Input: part model. Units: mm. Frame: model coordinates. Round coordinates to 2 decimals unless told otherwise and drop trailing zeros. Write each loop counter-clockwise with the first axis right and the second up, starting at its lowest first coordinate (ties: lowest second). Pieces come first, ordered by that corner, then holes. Notation, with made-up numbers: (-35, 16.25) -> (-22, 16.25) arc R20 ccw to (-22, 32.25) -> close; hole circle Ø7 at (10.5, -30.75). An arc over 180 degrees is marked (long way). Write item = value, one per line.
```python
from build123d import *

# Parameters (mm, degrees)
SKETCH1_R           = 2.1
BOSS_EXTRUDE1_DEPTH = 3


with BuildPart() as part:
    # Sketch1 → Boss-Extrude1 (new body)
    with BuildSketch(Plane(origin=(0, 0, 0), x_dir=(1, 0, 0), z_dir=(0, 1, 0))):
        with BuildLine():
            Line((65, -70), (-65, -70))
            ThreePointArc((-65, -70), (-98.297426292, -61.573382255), (-123.578147349, -38.32232578))
            Line((-123.578147349, -38.32232578), (-67.663660863, -38.32232578))
            Line((-67.663660863, -38.32232578), (-67.663660863, 37.858201233))
            Line((-67.663660863, 37.858201233), (-123.879169486, 37.858201233))
            ThreePointArc((-123.879169486, 37.858201233), (-98.540467451, 61.441330089), (-65, 70))
            Line((-65, 70), (65, 70))
            Line((65, 70), (65, -70))
        make_face()
        with Locations((-44.999784569, 59.999822317)):
            Circle(SKETCH1_R, mode=Mode.SUBTRACT)
        with Locations((-44.999784569, -60.000177683)):
            Circle(SKETCH1_R, mode=Mode.SUBTRACT)
        with Locations((55.000215431, 59.999822317)):
            Circle(SKETCH1_R, mode=Mode.SUBTRACT)
        with Locations((55.000215431, -60.000177683)):
            Circle(SKETCH1_R, mode=Mode.SUBTRACT)
    extrude(amount=BOSS_EXTRUDE1_DEPTH)


solid = part.part
```
1) Cut plane C-C (z = 0.5). Return the cut outline in (x, y).
Solutions:
outline = (-67.66, 0) -> (65, 0) -> (65, 3) -> (-67.66, 3) -> close
2) Draft query along Z for faces 1 (the face through (-7, 3, -1)), 2 (the face through (-45.46, 1.48, -57.95)), 3 (the face through (-98.969, 1.479, -61.205)). Return one class per face: +Z half, -Z half, draft (parallel to the pull), parting line (faces both ways), or undercut.
Solutions:
face_1 = draft
face_2 = undercut
face_3 = -Z half
3) Line query: L1, parallel to X at y = 2.4, z = -8; L2, parallel to X at y = 1.2, z = -50. Output: solid intervals per line, ascending. Write a range as from..to.
Solutions:
L1 = -67.66..65
L2 = -113.99..65
4) Cut plane A-A (x = -108). Return the cut outline in (y, z).
Solutions:
outline = (0, -55.24) -> (3, -55.24) -> (3, -37.86) -> (0, -37.86) -> close; (0, 38.32) -> (3, 38.32) -> (3, 55.24) -> (0, 55.24) -> close
5) Cut plane B-B (y = 1.25). Return the cut outline in (x, z).
Solutions:
outline = (-123.88, -37.86) arc R70 ccw to (-65, -70) -> (65, -70) -> (65, 70) -> (-65, 70) arc R70 ccw to (-123.58, 38.32) -> (-67.66, 38.32) -> (-67.66, -37.86) -> close; hole circle Ø4.2 at (-45, -60); hole circle Ø4.2 at (-45, 60); hole circle Ø4.2 at (55, -60); hole circle Ø4.2 at (55, 60)
6) First-contact query: P1, Ø1, axis at y = 2, z = -53, coming from the -X side. Flat tip, straight axial feed; report the tip coordinate or a pass-through.
Solutions:
P1 = -111.3
